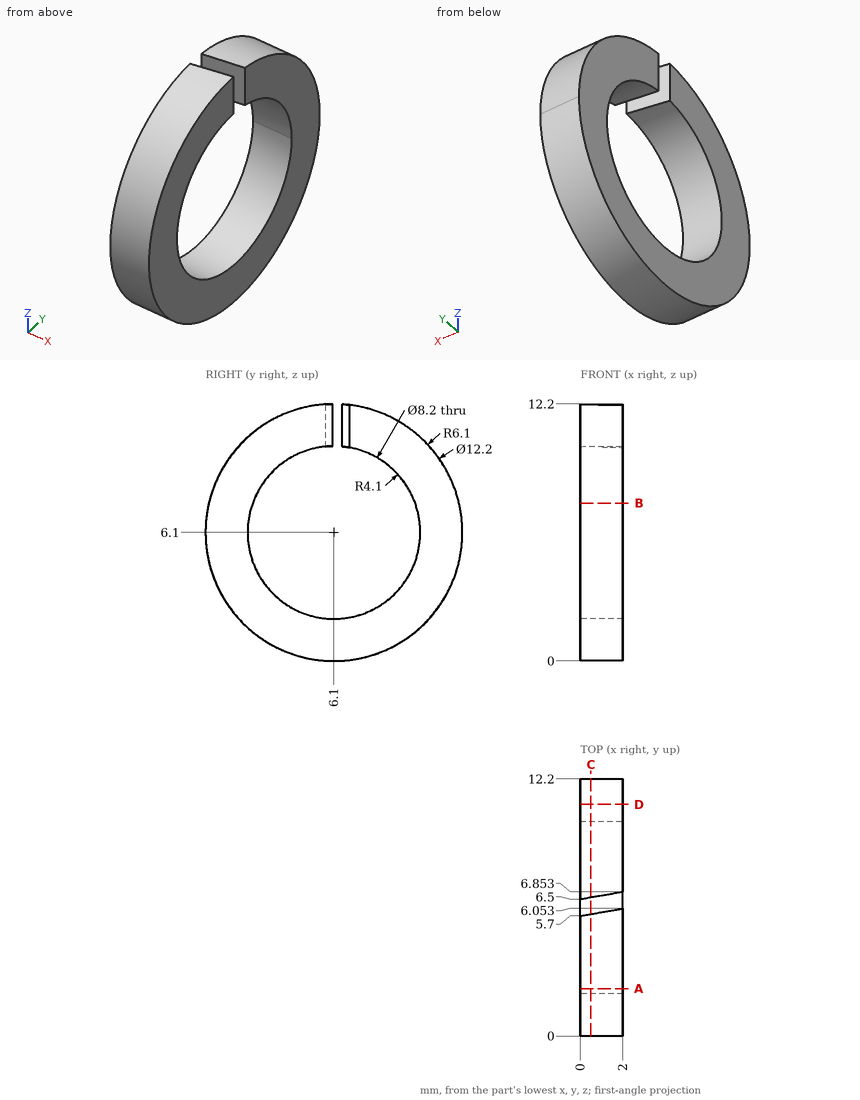
Could you check a few things on this drawing? It's one solid part, dimensions in mm from its lowest x, y, z. Give positions to 0.01 mm unless a question says otherwise; leave off trailing zeros. Write each loop counter-clockwise with the first axis right and the second up, starting at its lowest first coordinate (ties: lowest second). Pieces come first, ordered by that corner, then holes. Notation, with made-up numbers: (45.25, 52) -> (92.25, 52) arc R5 cw to (92.25, 61) -> close; hole circle Ø4 at (10, -9). An arc over 180 degrees is marked (long way). Write each question's results on one line, items separated by ' | '.
1. I want a section at A-A, the plane y = 2.25. Write out the boundary of the cut face in (x, z), then the cut area to 3 significant figures.
Check sheet entries:
outline: (0, 1.37) -> (2, 1.37) -> (2, 4.69) -> (0, 4.69) -> close; (0, 7.51) -> (2, 7.51) -> (2, 10.83) -> (0, 10.83) -> close | area: 13.3 mm²
2. Will this pin go through, and if not, where does the flat tip stop? pin 1 Ø6.5 at (y, z) = (6.1, 6.1) entering from -X.
Check sheet entries:
pin 1: passes through
3. I want a section at B-B, the plane z = 7.5. Write out the boundary of the cut face in (x, y).
Check sheet entries:
outline: (0, 0.16) -> (2, 0.16) -> (2, 2.25) -> (0, 2.25) -> close; (0, 9.95) -> (2, 9.95) -> (2, 12.04) -> (0, 12.04) -> close
4. I need wall thicknesses on L1, parallel to Y at x = 0.5, z = 6.1; L2, parallel to Z at x = 1.2, y = 6.1; L3, parallel to Z at x = 1.75, y = 7.75. Which ranges of each line are inside material? Lowest first, please.
Check sheet entries:
L1: y = 0 to 2, 10.2 to 12.2 | L2: z = 0 to 2 | L3: z = 0.23 to 2.35, 9.85 to 11.97
5. I want a section at D-D, the plane y = 11. Write out the boundary of the cut face in (x, z).
Check sheet entries:
outline: (0, 2.47) -> (2, 2.47) -> (2, 9.73) -> (0, 9.73) -> close
6. I want a section at C-C, the plane x = 0.5. Write out the boundary of the cut face in (y, z).
Check sheet entries:
outline: (5.79, 10.19) -> (5.79, 12.19) arc R6.1 ccw (long way) to (6.59, 12.18) -> (6.59, 10.17) arc R4.1 cw (long way) to start
